```python
from build123d import *

# Parameters (mm, degrees)
F0_R     = 44.711007
F1_DEPTH = 25
F3_R     = 30
F4_DEPTH = 50


with BuildPart() as f1:
    # F0 (on Front) → F1 (new body)
    with BuildSketch(Plane.XZ):
        Circle(F0_R)
    extrude(amount=F1_DEPTH)

    # F2: F1 across face


with BuildPart() as f1_1:
    add(f1.part)
    add(f1.part.mirror(Plane(origin=(0, 0, 0), x_dir=(1, 0, 0), z_dir=(0, 1, 0))))

    # F3 (on face) → F4 (cut)
    with BuildSketch(Plane.XZ.offset(25)):
        Circle(F3_R)
    extrude(amount=-F4_DEPTH, mode=Mode.SUBTRACT)


solid = f1_1.part
```
Source: CAD feature listing. Evaluate the final solid. Frame: model axes, mm. Round coordinates to 2 decimals unless told otherwise and drop trailing zeros. Write each loop counter-clockwise with the first axis right and the second up, starting at its lowest first coordinate (ties: lowest second). Pieces come first, ordered by that corner, then holes. Notation, with made-up numbers: M -0.75,17.5 L 24.25,17.5 A8 cw 24.25,29.5 Z; hole C -32.75,-24.75 d9. An arc over 180 degrees is marked long. Use CSV: the item, a comma, the result in double quotes. Start each with the question number.
Q1. Cut plane C-C on y = 18. Output: boundary loops of the cut face in (x, z), plus the area to 3 significant figures.
Q2. Cut plane A-A on x = 0. Output: boundary loops of the cut face in (y, z), plus the area to 3 significant figures.
Q3. Pull-direction query (X, two-part tool) for faces 1 (the face through (9, 25, -29)), 2 (the face through (-29.97, -0.35, 1.32)), 3 (the face through (-35.48, -0.35, -27.21)); classes: +X half, -X half, draft (parallel to the pull), parting line (faces both ways), or undercut.
Q4. Line query: line 1 (Z direction, x = 0, y = -5.5); line 2 (X direction, y = 18.5, z = -1); line 3 (X direction, y = -3.5, z = -13). Output: solid intervals per line, ascending. Write a range as from..to.
Q5. First-contact query: P1, Ø1.5, axis at y = 13, z = 32, coming from the -X side; P2, Ø5, axis at x = -12.5, y = -11, coming from the -Z side; P3, Ø2, axis at x = -28.5, y = 11.5, coming from the -Z side; P4, Ø10, axis at x = -17, z = -24.5, coming from the -Y side. Flat tips, straight axial feed; report the tip coordinate or a pass-through.
Q6. Cut plane D-D on x = 35. Output: boundary loops of the cut face in (y, z).
Q7. Cut plane B-B on z = -2.5. Output: boundary loops of the cut face in (x, y).
Results found:
1,outline,"C 0,0 d89.42; hole C 0,0 d60"
1,area,"3,450 mm^2"
2,outline,"M -25,-44.71 L 25,-44.71 L 25,-30 L -25,-30 Z; M -25,30 L 25,30 L 25,44.71 L -25,44.71 Z"
2,area,"1,470 mm^2"
3,face 1,"draft"
3,face 2,"undercut"
3,face 3,"parting line"
4,line 1,"-44.71..-30, 30..44.71"
4,line 2,"-44.7..-29.98, 29.98..44.7"
4,line 3,"-42.78..-27.04, 27.04..42.78"
5,P1,"x = -31.98"
5,P2,"z = -43.58"
5,P3,"z = -35.25"
5,P4,"y = -25"
6,outline,"M -25,-27.82 L 25,-27.82 L 25,27.82 L -25,27.82 Z"
7,outline,"M -44.64,-25 L -29.9,-25 L -29.9,25 L -44.64,25 Z; M 29.9,-25 L 44.64,-25 L 44.64,25 L 29.9,25 Z"
